```python
from build123d import *

# Parameters (mm, degrees)
F0_W     = 76.2
F0_H     = 76.2
F1_DEPTH = 7.62
F3_DEPTH = 6.35
F4_W     = 76.2
F4_H     = 76.2
F5_DEPTH = 25.4


with BuildPart() as f1:
    # F0 (on Front) → F1 (new body)
    with BuildSketch(Plane.XZ):
        with Locations((1.97351, -18.584051)):
            Rectangle(F0_W, F0_H)
    extrude(amount=F1_DEPTH)

    # F2 (on face) → F3 (cut)
    with BuildSketch(Plane.XZ.offset(7.62)):
        with BuildLine():
            ThreePointArc((-13.869856, -30.198783), (-23.613724, -33.018671), (-14.965154, -27.718014))
            Line((-14.965154, -27.718014), (-5.508855, -32.213487))
            Line((-5.508855, -32.213487), (15.947649, -42.256406))
            ThreePointArc((15.947649, -42.256406), (35.979187, -26.126775), (10.324704, -27.936473))
            Line((10.324704, -27.936473), (18.371095, -31.763075))
            ThreePointArc((18.371095, -31.763075), (27.571492, -28.044193), (21.199014, -35.651355))
            Line((21.199014, -35.651355), (9.986617, -30.198783))
            Line((9.986617, -30.198783), (7.381885, -28.932106))
            Line((7.381885, -28.932106), (14.229408, -15.111173))
            ThreePointArc((14.229408, -15.111173), (-3.707419, 3.005858), (-0.665507, -22.30626))
            Line((-0.665507, -22.30626), (2.75023, -14.190622))
            ThreePointArc((2.75023, -14.190622), (-1.129552, -5.110009), (6.792904, -11.004492))
            Line((6.792904, -11.004492), (2.213593, -22.604426))
            Line((2.213593, -22.604426), (0.713445, -25.689254))
            Line((0.713445, -25.689254), (-11.252215, -19.870372))
            ThreePointArc((-11.252215, -19.870372), (-31.530362, -35.752906), (-5.825069, -34.110951))
            Line((-5.825069, -34.110951), (-13.869856, -30.198783))
        make_face()
    extrude(amount=-F3_DEPTH, mode=Mode.SUBTRACT)

    # F4 (on face) → F5 (cut)
    with BuildSketch(Plane.XZ.offset(7.62)):
        with Locations((1.97351, -18.584051)):
            Rectangle(F4_W, F4_H)
        with BuildLine():
            ThreePointArc((-11.160331, -17.109246), (3.105819, 6.365386), (14.391984, -18.678653))
            ThreePointArc((14.391984, -18.678653), (38.724881, -29.989974), (16.189961, -44.557514))
            Line((16.189961, -44.557514), (-3.568678, -34.948918))
            ThreePointArc((-3.568678, -34.948918), (-33.539138, -37.167669), (-11.160331, -17.109246))
        make_face(mode=Mode.SUBTRACT)
    extrude(amount=-F5_DEPTH, mode=Mode.SUBTRACT)


solid = f1.part
```
Design review of the part built by this model. Coordinates are the model's own, in mm. A direction names the side the tool comes from. Round coordinates to 2 decimals unless told otherwise and drop trailing zeros. Order: outer loops, then holes, each group sorted by start corner. A loop starts at its lowest first (then second) coordinate and runs counter-clockwise, first axis right, second up. Notation, with made-up numbers: (72, 86) - (80, 86) arc R32 ccw to (80, 113) - close; hole circle Ø8 at (-24.5, 79). An arc over 180 degrees is marked (long way). One line per question, with ' | ' between items.
Item 1: Wall thickness on line 1 (X direction, y = -5, z = -9); line 2 (Z direction, x = -23, y = -3.75); line 3 (X direction, y = -7, z = -8): over which ranges is each line inside the solid? List them lowest first. Write a range as [from, to].
Checks:
line 1: [-13.37, -11.32], [-3.08, 7.15], [15.63, 17.68] | line 2: [-46.3, -43.81], [-34.06, -27.85], [-18.1, -15.61] | line 3: [-13.33, -11.27], [-2.95, 7.02], [15.58, 17.64]
Item 2: Draft analysis for pull direction X (two halves, no side actions). For faces 3 (the face through (1.47, -4.49, -24.13)), 4 (the face through (1, 0, -26)), 5 (the face through (6.45, -3.86, -39.82)), state which applies: +X half, -X half, draft (parallel to the pull), parting line (faces both ways), or undercut.
Checks:
face 3: undercut | face 4: draft | face 5: undercut
Item 3: Machinability: for faces 1 (the face through (-1, -7.62, -24)), 2 (the face through (-10.303, -4.489, -29.934)), which of the approach directions +Z, -Z, +X, -X, +Y, -Y give a long, thin tool a straight path to every point of the face, cutting with its end or side? Answer none if there is none.
Checks:
face 1: +Z, -Z, +X, -X, -Y | face 2: -Y
Item 4: Take a section at B-B, the plane x = 24. Write out the cut boundary in (y, z), then the cut area to 3 significant figures.
Checks:
outline: (-7.62, -46.37) - (0, -46.37) - (0, -15.74) - (-7.62, -15.74) - (-7.62, -17.59) - (-1.27, -17.59) - (-1.27, -25.97) - (-7.62, -25.97) - (-7.62, -36.14) - (-1.27, -36.14) - (-1.27, -44.52) - (-7.62, -44.52) - close | area: 127 mm²
Item 5: Take a section at D-D, the plane x = -28.5. Write out the cut boundary in (y, z).
Checks:
outline: (-7.62, -43.62) - (0, -43.62) - (0, -18.28) - (-7.62, -18.28) - (-7.62, -21.45) - (-1.27, -21.45) - (-1.27, -40.45) - (-7.62, -40.45) - close
Item 6: For P1, Ø5, axis at x = 19.5, z = -35, coming from the +Y side; P2, Ø3, axis at x = -3, y = -6.5, coming from the +Z side; P3, Ø2, axis at y = -5, z = -35.5, coming from the +X side; P4, Ø4, axis at y = -1, z = -2, coming from the +X side, all flat-tipped, find the tip position at first contact; note any pin that passes through.
Checks:
P1: y = 0 | P2: z = 5.96 | P3: x = 38.37 | P4: x = 16.81
Item 7: Take a section at A-A, the plane z = -8.5. Write out the cut boundary in (x, y), then the cut area to 3 significant figures.
Checks:
outline: (-13.36, -7.62) - (-11.31, -7.62) - (-11.31, -1.27) - (-3.04, -1.27) - (-3.04, -7.62) - (7.11, -7.62) - (7.11, -1.27) - (15.62, -1.27) - (15.62, -7.62) - (17.66, -7.62) - (17.66, 0) - (-13.36, 0) - close | area: 130 mm²
Item 8: Take a section at C-C, the plane y = -4. Write out the cut boundary in (x, z).
Checks:
outline: (-11.16, -17.11) arc R15.87 ccw (long way) to (-3.57, -34.95) - (16.19, -44.56) arc R15.33 ccw (long way) to (14.39, -18.68) arc R15.52 ccw (long way) to start; hole (-14.97, -27.72) - (-5.51, -32.21) - (15.95, -42.26) arc R13.48 ccw (long way) to (10.32, -27.94) - (18.37, -31.76) arc R5.11 cw (long way) to (21.2, -35.65) - (7.38, -28.93) - (14.23, -15.11) arc R13.48 ccw (long way) to (-0.67, -22.31) - (2.75, -14.19) arc R5.11 cw (long way) to (6.79, -11) - (2.21, -22.6) - (0.71, -25.69) - (-11.25, -19.87) arc R13.48 ccw (long way) to (-5.83, -34.11) - (-13.87, -30.2) arc R5.12 cw (long way) to start
